```python
from build123d import *

# Parameters (mm, degrees)
BOSS_EXTRUDE1_DEPTH = 20
SKETCH4_R           = 1.95
CUT_EXTRUDE1_DEPTH  = 20
BOSS_EXTRUDE2_DEPTH = 10
SKETCH8_W           = 12
SKETCH8_H           = 8
BOSS_EXTRUDE3_DEPTH = 5
CUT_EXTRUDE3_REACH  = 14


with BuildPart() as part:
    # Sketch2 → Boss-Extrude1 (new body)
    with BuildSketch(Plane(origin=(0, 0, 0), x_dir=(1, 0, 0), z_dir=(0, 1, 0))):
        Polygon((5.542562584, 0), (2.771281292, 4.8), (0.9, 4.8), (0.9, 5.75), (-0.9, 5.75), (-0.9, 4.8), (-2.771281292, 4.8), (-5.542562584, 0), (-2.771281292, -4.8), (2.771281292, -4.8), align=None)
    extrude(amount=BOSS_EXTRUDE1_DEPTH)

    # Sketch4 → Cut-Extrude1 (cut)
    with BuildSketch(Plane(origin=(0, 0, 0), x_dir=(-1, 0, 0), z_dir=(0, -1, 0))):
        Circle(SKETCH4_R)
    extrude(amount=-CUT_EXTRUDE1_DEPTH, mode=Mode.SUBTRACT)

    # Sketch6 → Boss-Extrude2 (add)
    with BuildSketch(Plane.XZ):
        Polygon((0.9, -5.75), (0.9, -11), (6, -11), (6, -19), (-6, -19), (-6, -11), (-0.9, -11), (-0.9, -5.75), align=None)
    extrude(amount=-BOSS_EXTRUDE2_DEPTH)

    # Sketch8 → Boss-Extrude3 (add)
    with BuildSketch(Plane(origin=(0, 0, 0), x_dir=(-1, 0, 0), z_dir=(0, -1, 0))):
        with Locations((0, 15)):
            Rectangle(SKETCH8_W, SKETCH8_H)
    extrude(amount=BOSS_EXTRUDE3_DEPTH)

    # Sketch9 → Cut-Extrude3 (cut, up to next)
    with BuildSketch(Plane(origin=(6, 0, 0), x_dir=(0, 0, -1), z_dir=(1, 0, 0)), mode=Mode.PRIVATE) as cut_extrude3_sk1:
        with BuildLine():
            Line((13, 10), (19, 10))
            Line((19, 10), (19, -3))
            ThreePointArc((19, -3), (15.413604557, 3.22935595), (13, 10))
        make_face()
    cut_extrude3_tool1 = extrude(cut_extrude3_sk1.sketch, amount=-CUT_EXTRUDE3_REACH, mode=Mode.PRIVATE) & part.part
    add(cut_extrude3_tool1.solids().sort_by_distance((6, 5.355709, -16.831232))[0], mode=Mode.SUBTRACT)


solid = part.part
```
Can you work these out from the model? Positions are in its coordinate system, mm. A direction names the side the tool comes from. Round coordinates to 2 decimals unless told otherwise and drop trailing zeros. Order: outer loops, then holes, each group sorted by start corner. A loop starts at its lowest first (then second) coordinate and runs counter-clockwise, first axis right, second up.
(1) If we section it at D-D (x = 1.5): Please give me the cut outline in (y, z), plus the area to 3 significant figures.
Results are:
outline: (-5, -19) - (-3, -19) arc R40 cw to (10, -13) - (10, -11) - (-5, -11) - close; (0, -4.8) - (20, -4.8) - (20, -1.25) - (0, -1.25) - close; (0, 1.25) - (20, 1.25) - (20, 4.8) - (0, 4.8) - close
area: 217 mm2
(2) If we section it at C-C (z = 1.25): Please give me the cut outline in (x, y).
Results are:
outline: (-4.82, 0) - (-1.5, 0) - (-1.5, 20) - (-4.82, 20) - close; (1.5, 0) - (4.82, 0) - (4.82, 20) - (1.5, 20) - close
(3) If we section it at B-B (y = 3.25): Please give me the cut outline in (x, z), plus the area to 3 significant figures.
Results are:
outline: (-6, -15.4) - (6, -15.4) - (6, -11) - (0.9, -11) - (0.9, -4.8) - (2.77, -4.8) - (5.54, 0) - (2.77, 4.8) - (-2.77, 4.8) - (-5.54, 0) - (-2.77, -4.8) - (-0.9, -4.8) - (-0.9, -11) - (-6, -11) - close; hole circle Ø3.9 at (0, 0)
area: 132 mm2
(4) I'm going to push flat-ended pins straight in: pin 1 (5 mm diameter, centred on x = 0, z = 0, fed in from -Y); pin 2 (8 mm diameter, centred on y = 9, z = -5.5, fed in from -X); pin 3 (2 mm diameter, centred on x = -4, y = 13, fed in from -Z); pin 4 (5 mm diameter, centred on x = 1.5, z = -7, fed in from +Y). Where does each tip first touch, or does it pass through?
Results are:
pin 1: stops at y = 0
pin 2: stops at x = -4.68
pin 3: stops at z = -4.4
pin 4: stops at y = 20
(5) On a 3-axis mill with a long thin cutter (end or side, diameter ignored), from which of +Z, -Z, +X, -X, +Y, -Y can I reach the whole of each face in a straight line? I mean faces 5 (the face through (0, 0, -3)), 6 (the face through (-2, 10, -4.8)), 7 (the face through (0, 15, -5.75)), 8 (the face through (2, 10, -4.8)). Say none if no direction works.
Results are:
face 5: +Z, +X, -X, -Y
face 6: -X, +Y, -Y
face 7: -Z, +X, -X, +Y
face 8: +X, +Y, -Y
(6) We'd pull the mould along Z, two halves only. Please class faces 1 (the face through (-1.2, 2.6, -11)), 2 (the face through (-4.176, 9.86, 2.366)), 3 (the face through (0.9, 5, -8)), 4 (the face through (0.084, 3.138, -15.456)): +Z half, -Z half, draft (parallel to the pull), parting line (faces both ways), or undercut.
Results are:
face 1: undercut
face 2: +Z half
face 3: undercut
face 4: -Z half
(7) If I drill on L1, parallel to Z at x = 0, y = 13.25; L2, parallel to Z at x = -0.5, y = 4.5; L3, parallel to Y at x = 0, z = -8.25, over which ranges is the centre line in solid material (lowest first)?
Results are:
L1: z = -5.75 to -1.95, 1.95 to 4.8
L2: z = -14.85 to -1.88, 1.88 to 4.8
L3: y = 0 to 10
(8) If we section it at A-A (x = 0): Please give me the cut outline in (y, z).
Results are:
outline: (-5, -19) - (-3, -19) arc R40 cw to (10, -13) - (10, -5.75) - (20, -5.75) - (20, -1.95) - (0, -1.95) - (0, -11) - (-5, -11) - close; (0, 1.95) - (20, 1.95) - (20, 4.8) - (0, 4.8) - close
